Source: CAD feature listing. Evaluate the final solid. Frame: model axes, mm. A direction names the side the tool comes from. Give positions to 0.01 mm unless a question says otherwise; leave off trailing zeros. Loops run counter-clockwise (first coordinate to the right, second up) from the corner with the lowest first, then second, coordinate; pieces in that order, holes last. Notation, with made-up numbers: M -10,-15.5 L 31,-15.5 A11 cw 31,-3.5 Z; hole C -35.5,9 d11. An arc over 180 degrees is marked long. Answer in a Markdown table with one row per item.
```python
from build123d import *

# Parameters (mm, degrees)
BOSS_EXTRUDE1_DEPTH            = 30
F_20_0MM_DOWEL_HOLE1_D         = 20
F_20_0MM_DOWEL_HOLE1_DEPTH     = 74.0791
F_20_0MM_DOWEL_HOLE1_TIP       = 6.00860619
M8X1_0_TAPPED_HOLE1_AT_2_COUNT = 2
M8X1_0_TAPPED_HOLE1_AT_2_PITCH = 18


with BuildPart() as part:
    # Sketch1 → Boss-Extrude1 (new body)
    with BuildSketch(Plane.XY):
        with BuildLine():
            Line((0, 0), (-39.807538051, 0))
            Line((-39.807538051, 0), (-39.807538051, 6))
            Line((-39.807538051, 6), (-25.192461949, 6))
            Line((-25.192461949, 6), (-18.400886991, 31.346502809))
            ThreePointArc((-18.400886991, 31.346502809), (0, 45.466), (18.400886991, 31.346502809))
            Line((18.400886991, 31.346502809), (25.192461949, 6))
            Line((25.192461949, 6), (39.807538051, 6))
            Line((39.807538051, 6), (39.807538051, 0))
            Line((39.807538051, 0), (0, 0))
        make_face()
    extrude(amount=BOSS_EXTRUDE1_DEPTH)

    # Ø20.0mm Dowel Hole1
    with Locations(Plane(origin=(0, 26.416, 30), x_dir=(1, 0, 0), z_dir=(0, 0, 1))):
        with Locations((0, 0)):
            Hole(F_20_0MM_DOWEL_HOLE1_D / 2, depth=F_20_0MM_DOWEL_HOLE1_DEPTH)
            with Locations((0, 0, -(F_20_0MM_DOWEL_HOLE1_DEPTH + F_20_0MM_DOWEL_HOLE1_TIP / 2))):  # 118° drill point
                Cone(0, F_20_0MM_DOWEL_HOLE1_D / 2, F_20_0MM_DOWEL_HOLE1_TIP, mode=Mode.SUBTRACT)

    # Sketch6 → M8x1.0 Tapped Hole1 (revolve, cut)
    with BuildSketch(Plane(origin=(-32.5, 6, 6), x_dir=(0, 0, 1), z_dir=(1, 0, 0))):
        Polygon((0, 0), (0, 21.103012167), (3.5, 19), (3.5, 0), align=None)
    m8x1_0_tapped_hole1 = revolve(axis=Axis((-32.5, 12.35, 6), (0, -1, 0)), mode=Mode.SUBTRACT)

    # M8x1.0 Tapped Hole1 at 2: M8x1.0 Tapped Hole1 ×2
    with Locations(*[(0, 0, i * M8X1_0_TAPPED_HOLE1_AT_2_PITCH) for i in range(1, M8X1_0_TAPPED_HOLE1_AT_2_COUNT)]):
        add(m8x1_0_tapped_hole1, mode=Mode.SUBTRACT)

    # Mirror1: M8x1.0 Tapped Hole1 across plane
    add(m8x1_0_tapped_hole1.mirror(Plane(origin=(0, 0, 0), x_dir=(0, 0, 1), z_dir=(1, 0, 0))), mode=Mode.SUBTRACT)

    # Mirror1 copy 1 sketch → Mirror1 copy 1 (revolve, cut)
    with BuildSketch(Plane(origin=(32.5, 6, 24), x_dir=(0, 0, 1), z_dir=(-1, 0, 0))):
        Polygon((0, 0), (0, -21.103012167), (3.5, -19), (3.5, 0), align=None)
    revolve(axis=Axis((32.5, 12.35, 24), (0, 1, 0)), mode=Mode.SUBTRACT)


solid = part.part
```
Q1. Ray query, probe 1 along X at (y, z) = (4.1, 24); probe 2 along Z at (x, y) = (-32.5, 2.6); probe 3 along X at (y, z) = (3, 26.5). Return the intervals inside material, ascending. Write a range as from..to.
Values follow:
| item | result |
|---|---|
| probe 1 | -39.81..-36, -29..29, 36..39.81 |
| probe 2 | 0..2.5, 9.5..20.5, 27.5..30 |
| probe 3 | -39.81..-34.95, -30.05..30.05, 34.95..39.81 |
Q2. Section query C-C (x = 32.5). Output: boundary loops of the cut face in (y, z).
Values follow:
| item | result |
|---|---|
| outline | M 0,0 L 6,0 L 6,2.5 L 0,2.5 Z; M 0,9.5 L 6,9.5 L 6,20.5 L 0,20.5 Z; M 0,27.5 L 6,27.5 L 6,30 L 0,30 Z |
Q3. Mould query, pull axis X, two halves, no side actions, for faces 3 (the flat face through (-33, 6, 15)), 4 (the cylindrical face through (-36, 3, 24)), 5 (the cylindrical face through (-0.349, 45.463, 14.79)). Classes: +X half, -X half, draft (parallel to the pull), parting line (faces both ways), or undercut.
Values follow:
| item | result |
|---|---|
| face 3 | draft |
| face 4 | undercut |
| face 5 | parting line |
Q4. Section query D-D (y = 21). Output: boundary loops of the cut face in (x, z).
Values follow:
| item | result |
|---|---|
| outline | M -21.17,0 L -8.41,0 L -8.41,30 L -21.17,30 Z; M 8.41,0 L 21.17,0 L 21.17,30 L 8.41,30 Z |
Q5. Section query A-A (x = 0). Output: boundary loops of the cut face in (y, z), plus the area to 3 significant figures.
Values follow:
| item | result |
|---|---|
| outline | M 0,0 L 16.42,0 L 16.42,30 L 0,30 Z; M 36.42,0 L 45.47,0 L 45.47,30 L 36.42,30 Z |
| area | 764 mm^2 |
Q6. Reachability of faces 1 (the flat face through (32, 6, 15)), 2 (the flat face through (1, 13, 0)) from +Z, -Z, +X, -X, +Y, -Y: full face, straight path, thin tool, end or side. Return the list, or none.
Values follow:
| item | result |
|---|---|
| face 1 | +Z, -Z, +X, +Y |
| face 2 | -Z, +X, -X, +Y, -Y |
Q7. Contact query for flat-ended pins moving along their axis: pin 1 Ø2 at (y, z) = (24.5, 9.5) entering from -X; pin 2 Ø10 at (y, z) = (30, 5) entering from +X; pin 3 Ø2 at (x, z) = (26.5, 6.5) entering from -Y; pin 4 Ø4 at (y, z) = (36, 22.5) entering from +X. Output: stop coordinate, or through.
Values follow:
| item | result |
|---|---|
| pin 1 | x = -20.5 |
| pin 2 | x = 20.1 |
| pin 3 | y = 0 |
| pin 4 | x = 17.48 |
Q8. Section query B-B (z = 5.25). Output: boundary loops of the cut face in (x, y).
Values follow:
| item | result |
|---|---|
| outline | M -39.81,0 L -35.92,0 L -35.92,6 L -39.81,6 Z; M -29.08,0 L 29.08,0 L 29.08,6 L 25.19,6 L 18.4,31.35 A19.05 ccw -18.4,31.35 L -25.19,6 L -29.08,6 Z; M 35.92,0 L 39.81,0 L 39.81,6 L 35.92,6 Z; hole C 0,26.42 d20 |
